Input: part model. Units: mm. Frame: model coordinates. Face numbers are marked on the shaded views. A direction names the side the tool comes from. Round coordinates to 2 decimals unless told otherwise and drop trailing zeros. Order: outer loops, then holes, each group sorted by start corner. A loop starts at its lowest first (then second) coordinate and runs counter-clockwise, first axis right, second up. Notation, with made-up numbers: (51.25, -4) -> (98.25, -4) arc R24 ccw to (98.25, 6) -> close; hole circle Ø5 at (89.5, 74). An arc over 180 degrees is marked (long way). Use a Markdown table: item, result.
from build123d import *

# Parameters (mm, degrees)
SKETCH_1_R          = 4
EXTRUDE_1_DEPTH     = 14
SKETCH_2_R          = 2.75
CUT_EXTRUDE_1_DEPTH = 37.66824239
SKETCH_3_R          = 2
CUT_EXTRUDE_2_DEPTH = 47.462457963
CUT_EXTRUDE_3_REACH = 43.228
SKETCH_4_W          = 1
SKETCH_4_H          = 8.631373033


with BuildPart() as part:
    # 草图1 → 凸台-拉伸1 (new body)
    with BuildSketch(Plane.XY):
        Polygon((21, 0), (-21, 0), (-21, 6), (-9, 6), (-9, 32.6), (9, 32.6), (9, 6), (21, 6), align=None)
        with Locations((0, 20)):
            Circle(SKETCH_1_R, mode=Mode.SUBTRACT)
    extrude(amount=EXTRUDE_1_DEPTH)

    # 草图2 → 切除-拉伸1 (cut, through all)
    with BuildSketch(Plane(origin=(0, 6, 0), x_dir=(1, 0, 0), z_dir=(0, 1, 0))):
        with Locations(Location((16, -7, 0), (0, 0, 270))):
            Circle(SKETCH_2_R)
        with Locations(Location((-16, -7, 0), (0, 0, 90))):
            Circle(SKETCH_2_R)
    extrude(amount=-CUT_EXTRUDE_1_DEPTH, mode=Mode.SUBTRACT)

    # 草图3 → 切除-拉伸2 (cut, through all)
    with BuildSketch(Plane.ZY.offset(9)):
        with Locations((7, 27.6)):
            Circle(SKETCH_3_R)
    extrude(amount=-CUT_EXTRUDE_2_DEPTH, mode=Mode.SUBTRACT)

    # 草图4 → 切除-拉伸3 (cut, up to next)
    with BuildSketch(Plane.XY.offset(14), mode=Mode.PRIVATE) as cut_extrude_3_sk1:
        with Locations((0, 28.284313484)):
            Rectangle(SKETCH_4_W, SKETCH_4_H)
    cut_extrude_3_tool1 = extrude(cut_extrude_3_sk1.sketch, amount=-CUT_EXTRUDE_3_REACH, mode=Mode.PRIVATE) & part.part
    add(cut_extrude_3_tool1.solids().sort_by_distance((0, 28.284313, 14))[0], mode=Mode.SUBTRACT)


solid = part.part
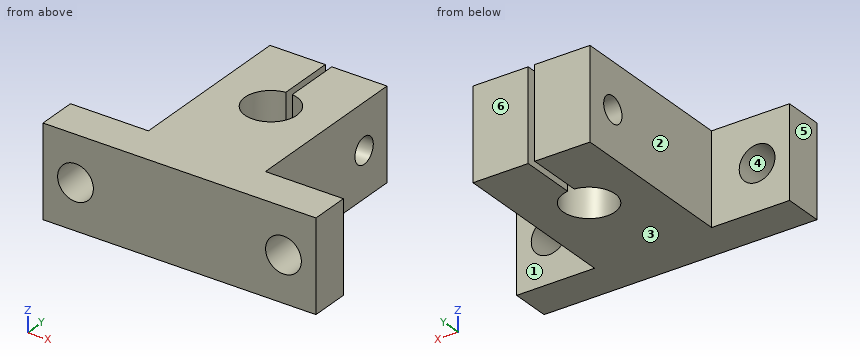
1) Ray query, probe 1 along X at (y, z) = (4.6, 7); probe 2 along X at (y, z) = (27.5, 10.5); probe 3 along Y at (x, z) = (4.25, 7). Return the intervals inside material, ascending.
Answer key:
| item | result |
|---|---|
| probe 1 | x = -21 to -18.75, -13.25 to 13.25, 18.75 to 21 |
| probe 2 | x = -9 to -0.5, 0.5 to 9 |
| probe 3 | y = 0 to 25.6, 29.6 to 32.6 |
2) Draft query along X for the marked faces 4, 5 and 6. Return one class per face: released by +X, released by -X, zero draft, split by the parting line, or undercut.
Answer key:
| item | result |
|---|---|
| face 4 | undercut |
| face 5 | released by -X |
| face 6 | zero draft |
3) Contact query for flat-ended pins moving along their axis: P1, Ø4.5, axis at y = 28.5, z = 8.5, coming from the +X side; P2, Ø2, axis at y = 19.5, z = 8.5, coming from the -X side; P3, Ø1.5, axis at x = -15, z = 11.5, coming from the +Y side. Output: stop coordinate, or through.
Answer key:
| item | result |
|---|---|
| P1 | stops at x = 9 |
| P2 | stops at x = -9 |
| P3 | stops at y = 6 |
4) Cut plane A-A on y = 25. Return loops of the section in (x, z), and give its area (3 significant figures).
Answer key:
| item | result |
|---|---|
| outline | (-9, 0) -> (-0.5, 0) -> (-0.5, 14) -> (-9, 14) -> close; (0.5, 0) -> (9, 0) -> (9, 14) -> (0.5, 14) -> close |
| area | 238 mm^2 |
5) Cut plane C-C on x = -16. Return loops of the section in (y, z), and give its area (3 significant figures).
Answer key:
| item | result |
|---|---|
| outline | (0, 0) -> (6, 0) -> (6, 4.25) -> (0, 4.25) -> close; (0, 9.75) -> (6, 9.75) -> (6, 14) -> (0, 14) -> close |
| area | 51.0 mm^2 |
6) Cut plane D-D on x = 1.5. Return loops of the section in (y, z).
Answer key:
| item | result |
|---|---|
| outline | (0, 0) -> (16.29, 0) -> (16.29, 14) -> (0, 14) -> close; (23.71, 0) -> (32.6, 0) -> (32.6, 14) -> (23.71, 14) -> close; hole circle Ø4 at (27.6, 7) |
7) Cut plane B-B on z = 7. Return loops of the section in (x, y).
Answer key:
| item | result |
|---|---|
| outline | (-21, 0) -> (-18.75, 0) -> (-18.75, 6) -> (-21, 6) -> close; (-13.25, 0) -> (13.25, 0) -> (13.25, 6) -> (9, 6) -> (9, 25.6) -> (0.5, 25.6) -> (0.5, 23.97) arc R4 cw (long way) to (-0.5, 23.97) -> (-0.5, 25.6) -> (-9, 25.6) -> (-9, 6) -> (-13.25, 6) -> close; (-9, 29.6) -> (-0.5, 29.6) -> (-0.5, 32.6) -> (-9, 32.6) -> close; (0.5, 29.6) -> (9, 29.6) -> (9, 32.6) -> (0.5, 32.6) -> close; (18.75, 0) -> (21, 0) -> (21, 6) -> (18.75, 6) -> close |
8) Set-up query: the marked faces 1, 2 and 3. Return all of +Z, -Z, +X, -X, +Y, -Y with unobstructed straight access to the full face (end or side cutting, diameter ignored); none if empty.
Answer key:
| item | result |
|---|---|
| face 1 | +Z, -Z, +X, +Y |
| face 2 | +Z, -Z, -X, +Y |
| face 3 | -Z, +X, -X, +Y, -Y |
